Part print with two shaded views. Sizes in mm from the minimum x, y, z corner. A direction names the side the tool comes from. Give positions to 0.01 mm unless a question says otherwise; leave off trailing zeros. Order: outer loops, then holes, each group sorted by start corner. A loop starts at its lowest first (then second) coordinate and runs counter-clockwise, first axis right, second up. Notation, with made-up numbers: M 7,21 L 26,21 A34 cw 26,60 Z; hole C 72,38 d11. An arc over 180 degrees is marked long. Answer as CSV lines item,"result".
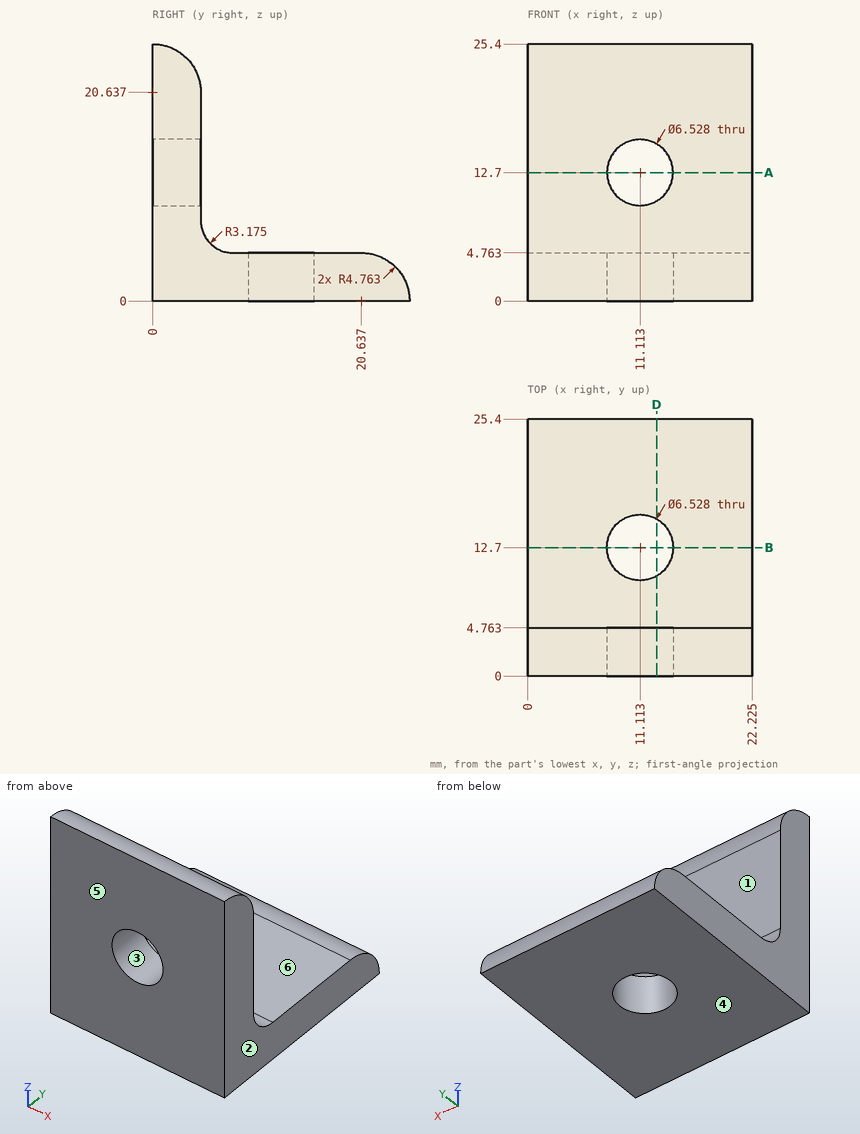
Item 1: Band-saw the part on D-D (x = 12.75). State how many separate pieces and enclosed holes the cut face has, and give its area (3 significant figures).
Geometry says:
separate pieces,"3"
enclosed holes,"0"
area,"158 mm2"
Item 2: Band-saw the part on A-A (z = 12.7). Give the cut face in (x, y) (1 decimal).
Geometry says:
outline,"M 0,0 L 7.8,0 L 7.8,4.8 L 0,4.8 Z; M 14.4,0 L 22.2,0 L 22.2,4.8 L 14.4,4.8 Z"
Item 3: Probe line 1 along X through (y, z) = (2.9, 12.7) (1 decimal); line 2 along X through (y, z) = (12.5, 4.25) (1 decimal); line 3 along Y through (x, z) = (20.5, 11.5). List the from-to ranges inside material, lowest first. Write a range as from..to.
Geometry says:
line 1,"x = 0..7.8, 14.4..22.2"
line 2,"x = 0..7.9, 14.4..22.2"
line 3,"y = 0..4.76"
Item 4: Pull direction Z, two halves, no side cores. Call the marked faces 3, 4, 5 and 6: released by +Z, released by -Z, zero draft, split by the parting line, or undercut.
Geometry says:
face 3,"undercut"
face 4,"released by -Z"
face 5,"zero draft"
face 6,"released by +Z"
Item 5: 3-axis set-ups, long thin cutter, end or side, ignore diameter. For the marked faces 1 and 2: which of +Z, -Z, +X, -X, +Y, -Y reach the whole face in a straight line?
Geometry says:
face 1,"+Z, +X, -X, +Y"
face 2,"+Z, -Z, +X, +Y, -Y"
Item 6: Drop a flat-ended pin along its axis: pin 1 (4 mm diameter, centred on x = 4.5, z = 14.5, fed in from +Y). Give the stop position or say it passes through.
Geometry says:
pin 1,"stops at y = 4.76"
